For this review, use the dimensioned drawing (mm, ordinates from the lowest corner) and the shaded views. A direction names the side the tool comes from. Give positions to 0.01 mm unless a question says otherwise; leave off trailing zeros. Write each loop counter-clockwise with the first axis right and the second up, starting at its lowest first coordinate (ties: lowest second). Pieces come first, ordered by that corner, then holes. Notation, with made-up numbers: M -5,-5 L 39,-5 A31 cw 39,27 Z; hole C 38.25,18 d2. An arc over 180 degrees is marked long. Write each question's results on one line, items separated by ' | '. Start each with the question number.
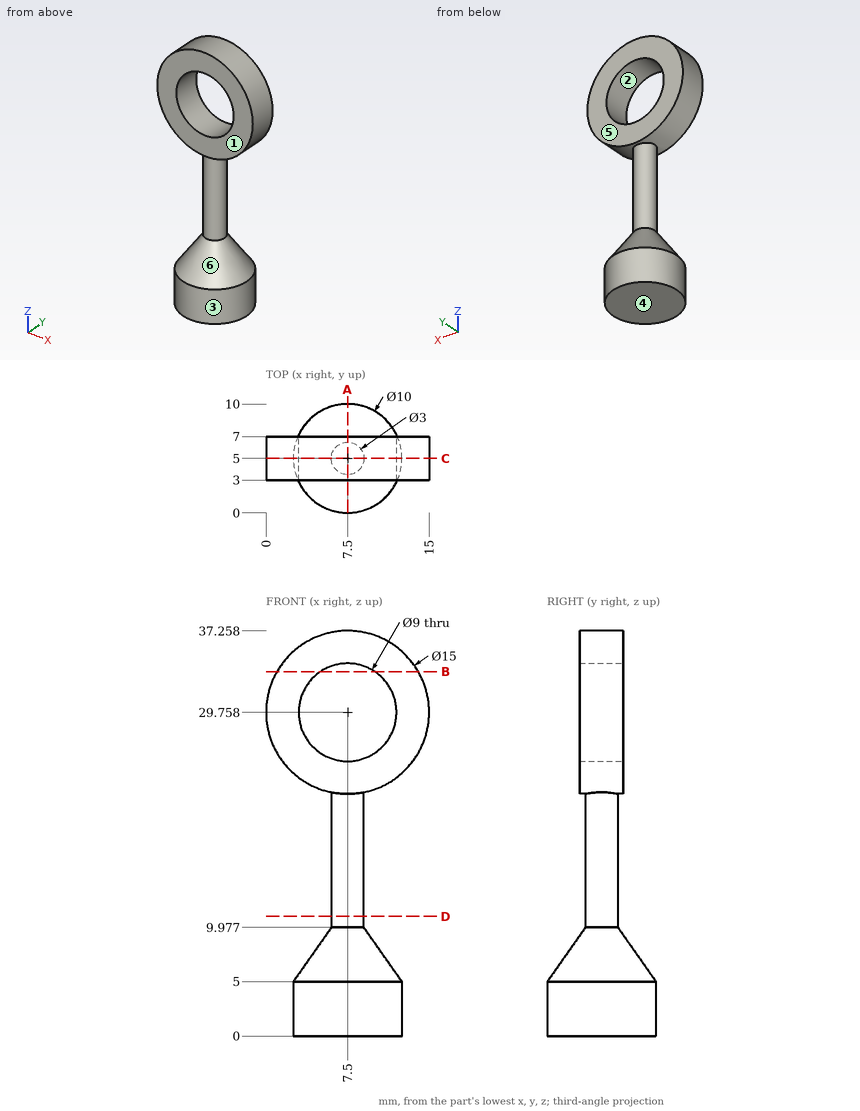
(1) Add section D-D (z = 11). State the section outline as (x, y) points.
(2) Wall thickness on L1, parallel to Z at x = 7.5, y = 4.05; L2, parallel to Z at x = 8.5, y = 8 (1 decimal); L3, parallel to Z at x = 3.75, y = 2.75: over which ranges is each line inside the solid? List them lowest first.
(3) Add section B-B (z = 33.5). State the section outline as (x, y) points, then the cut area to 3 significant figures.
(4) Add section C-C (y = 5). State the section outline as (x, z) points.
(5) Draft analysis for pull direction X (two halves, no side actions). For the marked faces 1, 2 and 3, state which applies: pulls with the +X half, pulls with the -X half, needs draft (parallel to the pull), parting line crosses it, or undercut.
(6) Add section A-A (x = 7.5). State the section outline as (y, z) points.
(7) Machinability: for the marked faces 4, 5 and 6, which of the approach directions +Z, -Z, +X, -X, +Y, -Y give a long, thin tool a straight path to every point of the face, cutting with its end or side? Answer none if there is none.
(8) Clearance check with flat-ended pins moving along their axes: P1, Ø8, axis at x = 7.5, z = 29.76, coming from the +Y side; P2, Ø2, axis at x = 8.5, z = 15.5, coming from the -Y side; P3, Ø3, axis at y = 3.5, z = 17, coming from the -X side; P4, Ø6, axis at x = 6, z = 26.5, coming from the -Y side. State where each tip first meets the part, or that it passes through.
Calculated:
1) outline: C 7.5,5 d3
2) L1: z = 0 to 25.26, 34.26 to 37.26 | L2: z = 0 to 7.6 | L3: z = 0 to 5.89
3) outline: M 1,3 L 5,3 L 5,7 L 1,7 Z; M 10,3 L 14,3 L 14,7 L 10,7 Z | area: 32.0 mm²
4) outline: M 2.5,0 L 12.5,0 L 12.5,5 L 9,9.98 L 9,22.41 A7.5 ccw long 6,22.41 L 6,9.98 L 2.5,5 Z; hole C 7.5,29.76 d9
5) face 1: needs draft | face 2: undercut | face 3: parting line crosses it
6) outline: M 0,0 L 10,0 L 10,5 L 6.5,9.98 L 6.5,22.26 L 7,22.26 L 7,25.26 L 3,25.26 L 3,22.26 L 3.5,22.26 L 3.5,9.98 L 0,5 Z; M 3,34.26 L 7,34.26 L 7,37.26 L 3,37.26 Z
7) face 4: -Z, +X, -X, +Y, -Y | face 5: +Z, +X, -X, +Y | face 6: none
8) P1: passes through | P2: stops at y = 3.5 | P3: stops at x = 6 | P4: stops at y = 3
